from build123d import *

# Parameters (mm, degrees)
SKETCH001_R                          = 4
SKETCH001_R_2                        = 1.6
EXTRUDE001_DEPTH                     = 12
SKETCH002_AS_DRAWN_W                 = 90
SKETCH002_AS_DRAWN_H                 = 30
SKETCH002_AS_DRAWN_R                 = 2.5
SKETCH002_AS_DRAWN_R_2               = 1.85
SKETCH002_AS_DRAWN_R_3               = 3.25
EXTRUDE002_DEPTH                     = 4
EXTRUDE002_ONTO_SKETCH002_ROLL_ANGLE = 90
SKETCH_R                             = 1.9
SKETCH_R_2                           = 12
SKETCH_R_3                           = 25
EXTRUDE_DEPTH                        = 3


with BuildPart() as extrude001:
    # Sketch001 → Extrude001 (new body)
    with BuildSketch(Plane.XY):
        with Locations((-50.5, -81)):
            Circle(SKETCH001_R)
        with Locations((-50.5, -81)):
            Circle(SKETCH001_R_2, mode=Mode.SUBTRACT)
        with Locations((50.5, -63)):
            Circle(SKETCH001_R)
        with Locations((50.5, -63)):
            Circle(SKETCH001_R_2, mode=Mode.SUBTRACT)
        with Locations((-50.5, 81)):
            Circle(SKETCH001_R)
        with Locations((-50.5, 81)):
            Circle(SKETCH001_R_2, mode=Mode.SUBTRACT)
        with Locations((50.5, 81)):
            Circle(SKETCH001_R)
        with Locations((50.5, 81)):
            Circle(SKETCH001_R_2, mode=Mode.SUBTRACT)
    extrude(amount=EXTRUDE001_DEPTH)


with BuildPart() as extrude002:
    # Sketch002 as drawn → Extrude002 (new)
    with BuildSketch(Plane.XY):
        with Locations((0, 15)):
            Rectangle(SKETCH002_AS_DRAWN_W, SKETCH002_AS_DRAWN_H)
        with Locations((-40, 9)):
            Circle(SKETCH002_AS_DRAWN_R, mode=Mode.SUBTRACT)
        with Locations((-40, 22)):
            Circle(SKETCH002_AS_DRAWN_R, mode=Mode.SUBTRACT)
        with Locations((-8, 22)):
            Circle(SKETCH002_AS_DRAWN_R, mode=Mode.SUBTRACT)
        with Locations((-8, 9)):
            Circle(SKETCH002_AS_DRAWN_R, mode=Mode.SUBTRACT)
        with Locations((7, 21)):
            Circle(SKETCH002_AS_DRAWN_R_2, mode=Mode.SUBTRACT)
        with Locations((28, 21)):
            Circle(SKETCH002_AS_DRAWN_R_2, mode=Mode.SUBTRACT)
        with Locations((7, 9)):
            Circle(SKETCH002_AS_DRAWN_R_2, mode=Mode.SUBTRACT)
        with Locations((28, 9)):
            Circle(SKETCH002_AS_DRAWN_R_2, mode=Mode.SUBTRACT)
        with Locations((37, 21)):
            Circle(SKETCH002_AS_DRAWN_R_3, mode=Mode.SUBTRACT)
    extrude(amount=-EXTRUDE002_DEPTH)


with BuildPart() as extrude002_1:
    # Extrude002 onto Sketch002 roll: moved
    add(extrude002.part.rotate(Axis((0, 0, 0), (1, 0, 0)), EXTRUDE002_ONTO_SKETCH002_ROLL_ANGLE))


with BuildPart() as extrude002_2:
    # Extrude002 onto Sketch002 placement: moved
    add(extrude002_1.part)


with BuildPart() as extrude002_3:
    # Extrude002 placement: moved
    add(extrude002_2.part.moved(Location((0, -105, 0))))


with BuildPart() as fusion:
    # Sketch → Extrude (new body)
    with BuildSketch(Plane.XY):
        Polygon((-55, 85), (55, 85), (55, -85), (45, -105), (-45, -105), (-55, -85), align=None)
        with Locations((-50.5, -81)):
            Circle(SKETCH_R, mode=Mode.SUBTRACT)
        with Locations((50.5, -63)):
            Circle(SKETCH_R, mode=Mode.SUBTRACT)
        with Locations((50.5, 81)):
            Circle(SKETCH_R, mode=Mode.SUBTRACT)
        with Locations((-50.5, 81)):
            Circle(SKETCH_R, mode=Mode.SUBTRACT)
        with Locations((-30, 40)):
            Circle(SKETCH_R_2, mode=Mode.SUBTRACT)
        with Locations((30, 40)):
            Circle(SKETCH_R_2, mode=Mode.SUBTRACT)
        with Locations((30, -40)):
            Circle(SKETCH_R_2, mode=Mode.SUBTRACT)
        with Locations((-30, -40)):
            Circle(SKETCH_R_2, mode=Mode.SUBTRACT)
        Circle(SKETCH_R_3, mode=Mode.SUBTRACT)
        with BuildLine():
            ThreePointArc((-40, -89), (-45.75, -94.75), (-40, -100.5))
            Line((-40, -100.5), (-37, -100.5))
            ThreePointArc((-37, -100.5), (-31.25, -94.75), (-37, -89))
            Line((-40, -89), (-37, -89))
        make_face(mode=Mode.SUBTRACT)
        with BuildLine():
            ThreePointArc((-11, -89), (-16.75, -94.75), (-11, -100.5))
            Line((-11, -100.5), (-8, -100.5))
            ThreePointArc((-8, -100.5), (-2.25, -94.75), (-8, -89))
            Line((-11, -89), (-8, -89))
        make_face(mode=Mode.SUBTRACT)
    extrude(amount=EXTRUDE_DEPTH)

    # Fusion: union Extrude001, Extrude002
    add(extrude001.part)
    add(extrude002_3.part)


solid = fusion.part
Could you check a few things on this model? Use its own coordinates, in mm. A direction names the side the tool comes from. Coordinates: 2 decimals unless noted, no trailing zeros. Order: outer loops, then holes, each group sorted by start corner. A loop starts at its lowest first (then second) coordinate and runs counter-clockwise, first axis right, second up.
Q1. Suppose I cut it at A-A on y = 36.5. Please give me the cut outline in (x, z), and give its area (3 significant figures).
Q2. Suppose I cut it at D-D on y = -94.75. Please give me the cut outline in (x, z) (3 decimals), and give its area (3 significant figures).
Q3. Thinking about a two-plate mould opening in Z: for faces 4 (the cylindrical face through (26.15, -103.03, 9.08)), 5 (the cylindrical face through (-51.367, 77.095, 7.437)), 6 (the flat face through (50, -65, 12)), which applies, released by +Z, released by -Z, zero draft, split by the parting line, or undercut?
Q4. Suppose I cut it at B-B on x = 37. Please give me the cut outline in (y, z), and give its area (3 significant figures).
Q5. Will these pins go through, and if not, where does the flat tip stop? pin 1 (3 mm diameter, centred on x = 28, z = 9, fed in from +Y); pin 2 (8 mm diameter, centred on x = 5.5, z = 9, fed in from -Y); pin 3 (2 mm diameter, centred on x = 34, y = 8, fed in from +Z); pin 4 (2 mm diameter, centred on x = 21, z = 7.5, fed in from +Y).
Q6. Suppose I cut it at C-C on y = 12.5. Please give me the cut outline in (x, z).
Q7. Please list where these lines run through material, in increasing order: L1, parallel to Y at x = 30, z = 1.1; L2, parallel to Z at x = -27, y = 68.5; L3, parallel to Y at x = -1, z = 10.
Q8. Which directions (+Z, -Z, +X, -X, +Y, -Y) give clear straight access to the entire face, cutting with the end or side of a thin tool? Please do faces 1 (the cylindrical face through (-8.54, -103.03, 6.56)), 2 (the cylindrical face through (-16.75, -94.62, 1.48)), 3 (the cylindrical face through (49.633, -66.905, 7.437)).
Answer:
1. outline: (-55, 0) - (-41.48, 0) - (-41.48, 3) - (-55, 3) - close; (-18.52, 0) - (18.52, 0) - (18.52, 3) - (-18.52, 3) - close; (41.48, 0) - (55, 0) - (55, 3) - (41.48, 3) - close
1. area: 192 mm2
2. outline: (-50.125, 0) - (-45.75, 0) - (-45.75, 3) - (-50.125, 3) - close; (-31.25, 0) - (-16.75, 0) - (-16.75, 3) - (-31.25, 3) - close; (-2.25, 0) - (50.125, 0) - (50.125, 3) - (-2.25, 3) - close
2. area: 214 mm2
3. face 4: undercut
3. face 5: zero draft
3. face 6: released by +Z
4. outline: (-105, 0) - (-49.75, 0) - (-49.75, 3) - (-101, 3) - (-101, 17.75) - (-105, 17.75) - close; (-105, 24.25) - (-101, 24.25) - (-101, 30) - (-105, 30) - close; (-30.25, 0) - (30.25, 0) - (30.25, 3) - (-30.25, 3) - close; (49.75, 0) - (85, 0) - (85, 3) - (49.75, 3) - close
4. area: 535 mm2
5. pin 1: passes through
5. pin 2: stops at y = -105
5. pin 3: stops at z = 3
5. pin 4: stops at y = -101
6. outline: (-55, 0) - (-21.65, 0) - (-21.65, 3) - (-55, 3) - close; (21.65, 0) - (55, 0) - (55, 3) - (21.65, 3) - close
7. L1: y = -105 to -52, -28 to 28, 52 to 85
7. L2: z = 0 to 3
7. L3: y = -105 to -101
8. face 1: +Y, -Y
8. face 2: +Z, -Z
8. face 3: +Z
